from build123d import *

# Parameters (mm, degrees)
BOSS_EXTRUDE1_DEPTH = 3
SKETCH2_W           = 6
SKETCH2_H           = 10
CUT_EXTRUDE1_DEPTH  = 141.491992654
SKETCH3_W           = 3
SKETCH3_H           = 20
SKETCH3_W_2         = 20
SKETCH3_H_2         = 10
SKETCH3_W_3         = 10
SKETCH3_H_3         = 5
SKETCH3_W_4         = 5
CUT_EXTRUDE2_DEPTH  = 141.491992654
SKETCH4_W           = 5
SKETCH4_H           = 25
CUT_EXTRUDE3_DEPTH  = 141.491992654


with BuildPart() as part:
    # Sketch1 → Boss-Extrude1 (new body)
    with BuildSketch(Plane.XY):
        Polygon((0, 0), (47, 0), (47, -6), (77, -6), (77, 0), (124, 0), (124, 15), (127, 15), (127, 45), (124, 45), (124, 60), (0, 60), (0, 45), (-3, 45), (-3, 15), (0, 15), align=None)
    extrude(amount=BOSS_EXTRUDE1_DEPTH)

    # Sketch2 → Cut-Extrude1 (cut, through all)
    with BuildSketch(Plane.XY.offset(3)):
        with Locations((3, 55)):
            Rectangle(SKETCH2_W, SKETCH2_H)
        with Locations((121, 55)):
            Rectangle(SKETCH2_W, SKETCH2_H)
    extrude(amount=-CUT_EXTRUDE1_DEPTH, mode=Mode.SUBTRACT)

    # Sketch3 → Cut-Extrude2 (cut, through all)
    with BuildSketch(Plane.XY.offset(3)):
        Polygon((54.5, 57), (69.5, 57), (69.5, 54), (72, 54), (72, 49), (52, 49), (52, 54), (54.5, 54), align=None)
        with Locations((38, 24)):
            Rectangle(SKETCH3_W, SKETCH3_H)
        with Locations((86, 24)):
            Rectangle(SKETCH3_W, SKETCH3_H)
        with Locations((62, 24)):
            Rectangle(SKETCH3_W_2, SKETCH3_H_2)
        with Locations((48.5, 6.5)):
            Rectangle(SKETCH3_W_3, SKETCH3_H_3)
        with Locations((77.5, 23.5)):
            Rectangle(SKETCH3_W_4, SKETCH3_H_3)
    extrude(amount=-CUT_EXTRUDE2_DEPTH, mode=Mode.SUBTRACT)

    # Sketch4 → Cut-Extrude3 (cut, through all)
    with BuildSketch(Plane.XY.offset(3)):
        with Locations((16.5, 30)):
            Rectangle(SKETCH4_W, SKETCH4_H)
        with Locations((107.5, 30)):
            Rectangle(SKETCH4_W, SKETCH4_H)
    extrude(amount=-CUT_EXTRUDE3_DEPTH, mode=Mode.SUBTRACT)


solid = part.part
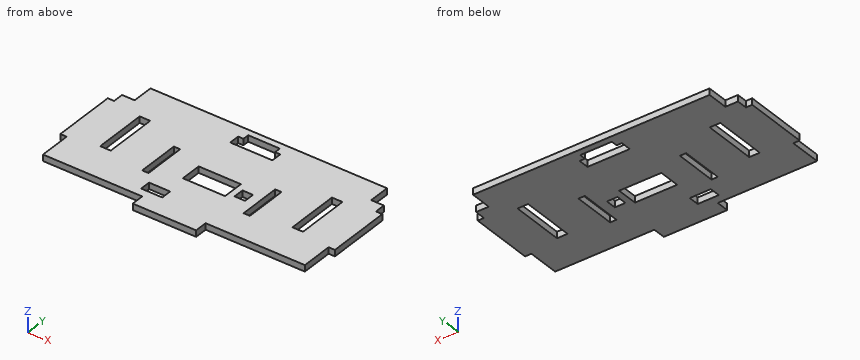
Here's how the part is built. I have some questions about the finished solid (model axes, mm). Coordinates: 2 decimals unless noted, no trailing zeros. Loops run counter-clockwise (first coordinate to the right, second up) from the corner with the lowest first, then second, coordinate; pieces in that order, holes last. Notation, with made-up numbers: (16.5, -9.5) -> (67.5, -9.5) arc R15 ccw to (67.5, 7.5) -> close; hole circle Ø1 at (4, 72.5). An arc over 180 degrees is marked (long way). Use one line per item in the form item = value. Start each with the question number.
(1) If we section it at A-A (y = 30.5): Please give me the cut outline in (x, z), then the cut area to 3 significant figures.
(2) Will these pins go through, and if not, where does the flat tip stop? pin 1 (0.9 mm diameter, centred on x = 17.5, z = 2, fed in from -Y); pin 2 (0.9 mm diameter, centred on y = 55, z = 1.5, fed in from -X).
(3) If we section it at D-D (y = 52.5): Please give me the cut outline in (x, z), then the cut area to 3 significant figures.
(4) If we section it at B-B (x = 62): Please give me the cut outline in (y, z).
(5) If we section it at C-C (y = 39.5): Please give me the cut outline in (x, z).
(6) Please list where these lines run through material, in increasing order: line 1 along X through (y, z) = (28.5, 0.6); line 2 along X through (y, z) = (32, 2.75); line 3 along X through (y, z) = (14.5, 1.65).
Verdict:
q1.outline = (-3, 0) -> (14, 0) -> (14, 3) -> (-3, 3) -> close; (19, 0) -> (36.5, 0) -> (36.5, 3) -> (19, 3) -> close; (39.5, 0) -> (84.5, 0) -> (84.5, 3) -> (39.5, 3) -> close; (87.5, 0) -> (105, 0) -> (105, 3) -> (87.5, 3) -> close; (110, 0) -> (127, 0) -> (127, 3) -> (110, 3) -> close
q1.area = 342 mm²
q2.pin_1 = 0
q2.pin_2 = 6
q3.outline = (6, 0) -> (52, 0) -> (52, 3) -> (6, 3) -> close; (72, 0) -> (118, 0) -> (118, 3) -> (72, 3) -> close
q3.area = 276 mm²
q4.outline = (-6, 0) -> (19, 0) -> (19, 3) -> (-6, 3) -> close; (29, 0) -> (49, 0) -> (49, 3) -> (29, 3) -> close; (57, 0) -> (60, 0) -> (60, 3) -> (57, 3) -> close
q5.outline = (-3, 0) -> (14, 0) -> (14, 3) -> (-3, 3) -> close; (19, 0) -> (105, 0) -> (105, 3) -> (19, 3) -> close; (110, 0) -> (127, 0) -> (127, 3) -> (110, 3) -> close
q6.line_1 = -3 to 14, 19 to 36.5, 39.5 to 52, 72 to 84.5, 87.5 to 105, 110 to 127
q6.line_2 = -3 to 14, 19 to 36.5, 39.5 to 84.5, 87.5 to 105, 110 to 127
q6.line_3 = 0 to 36.5, 39.5 to 84.5, 87.5 to 124
